```python
from build123d import *

# Parameters (mm, degrees)
F0_R     = 11.075
F1_DEPTH = 7
F2_SIZE2 = 6
F2_SIZE  = 3.5
F3_SIZE2 = 3.49999
F3_SIZE  = 5.99999
F4_SIZE  = 1.5


# Not quite as in the source:
# - a fillet or chamfer is up to 0.001 mm smaller than in the source, because OpenCascade refuses the exact size


with BuildPart() as f1:
    # F0 (on Top) → F1 (new body)
    with BuildSketch(Plane.XY):
        with BuildLine():
            ThreePointArc((28.2842712475, -28.2842712475), (21.9994915516, 0), (28.2842712475, 28.2842712475))
            ThreePointArc((28.2842712475, 28.2842712475), (0, 21.9994915516), (-28.2842712475, 28.2842712475))
            ThreePointArc((-28.2842712475, 28.2842712475), (-21.9994915516, 0), (-28.2842712475, -28.2842712475))
            ThreePointArc((-28.2842712475, -28.2842712475), (0, -21.9994915516), (28.2842712475, -28.2842712475))
        make_face()
        Circle(F0_R, mode=Mode.SUBTRACT)
    extrude(amount=F1_DEPTH)

    # F2
    f2_edges = [f1.edges().sort_by_distance(p)[0] for p in [
        (0, -21.999492, 7),
        (-21.999492, 0, 7),
        (0, 21.999492, 7),
        (21.999492, 0, 7),
    ]]
    chamfer(f2_edges, length=F2_SIZE, length2=F2_SIZE2)

    # F3 (size 6 and 3.5 in the source; OpenCascade refuses exactly that, so slightly less here)
    f3_edges = [f1.edges().sort_by_distance(p)[0] for p in [
        (-21.999492, 0, 0),
        (0, -21.999492, 0),
        (21.999492, 0, 0),
        (0, 21.999492, 0),
    ]]
    f3_side = f1.faces().sort_by_distance((0, -21.199492, 0))[0]
    chamfer(f3_edges, length=F3_SIZE, length2=F3_SIZE2, reference=f3_side)

    # F4
    f4_edges = [f1.edges().sort_by_distance(p)[0] for p in [
        (-11.075, 0, 0),
        (-11.075, 0, 7),
    ]]
    chamfer(f4_edges, length=F4_SIZE)


solid = f1.part
```
Build history of the part. All positions in model axes, mm. Give positions to 0.01 mm unless a question says otherwise; leave off trailing zeros. Loops run counter-clockwise (first coordinate to the right, second up) from the corner with the lowest first, then second, coordinate; pieces in that order, holes last.
1) Two-plate mould, pull along Y, no slides. Class faces 1 (the face through (0.42, 20.29, 4.5)), 2 (the face through (-20.376, 0.419, 2.552)), 3 (the face through (12, 4.3, 0)): released by +Y, released by -Y, zero draft, split by the parting line, or undercut.
Values follow:
face 1: released by +Y
face 2: undercut
face 3: zero draft
2) Probe line 1 along Y through (x, z) = (0, 2.95) (3 decimals); line 2 along X through (y, z) = (9, 1.5); line 3 along X through (y, z) = (-7, 1). List the from-to ranges inside material, lowest first.
Values follow:
line 1: y = -21.057 to -11.075, 11.075 to 21.057
line 2: x = -19.15 to -6.45, 6.45 to 19.15
line 3: x = -18.06 to -9.22, 9.22 to 18.06
3) Drop flat-ended pins along their axis: P1, Ø3, axis at y = -3.5, z = 5.5, coming from the -X side; P2, Ø6, axis at x = -20.5, y = -4, coming from the +Z side; P3, Ø3, axis at y = -0.5, z = 1, coming from the +X side. Give the stop position or say it passes through.
Values follow:
P1: stops at x = -21.23
P2: stops at z = 6.19
P3: stops at x = 20.29
4) Band-saw the part on C-C on z = 4.75. List the corners of the cut face in (x, y) (3 decimals), then the cut area to 3 significant figures.
Values follow:
outline: (-24.271, -24.271) arc R68.931 cw to (24.271, -24.271) arc R68.931 cw to (24.271, 24.271) arc R68.931 cw to (-24.271, 24.271) arc R68.931 cw to start; hole circle Ø22.15 at (0, 0)
area: 1,400 mm2
